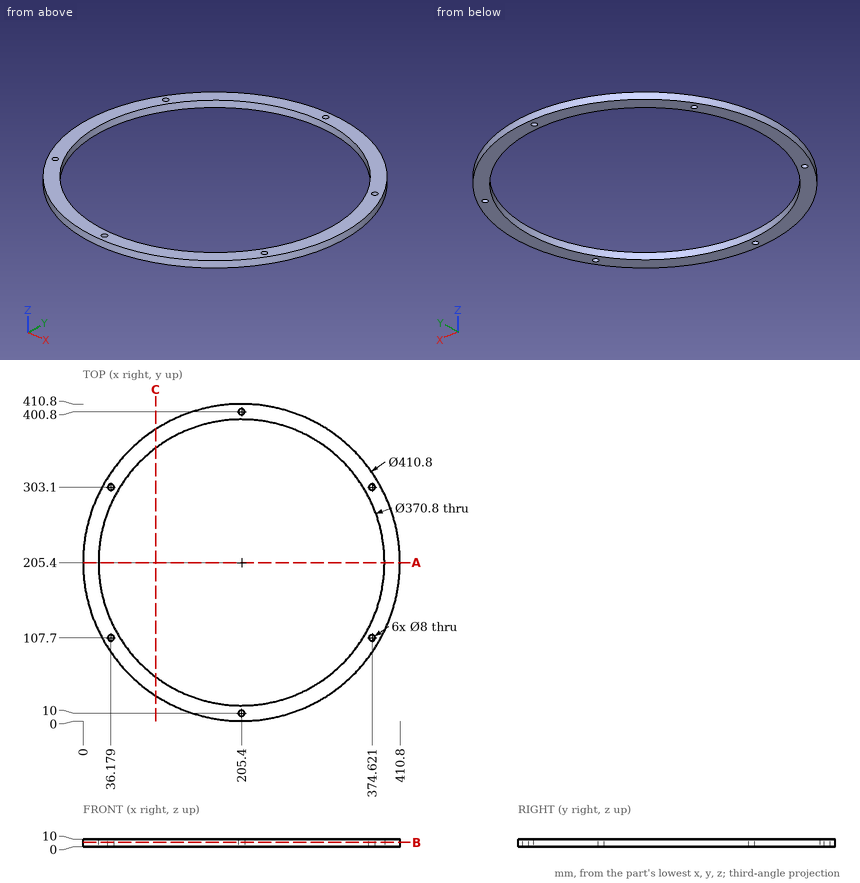
Drawing for the job (mm, zero at the part's lowest x, y, z). Round coordinates to 2 decimals unless told otherwise and drop trailing zeros. Order: outer loops, then holes, each group sorted by start corner. A loop starts at its lowest first (then second) coordinate and runs counter-clockwise, first axis right, second up. Notation, with made-up numbers: (-3.75, -15) -> (1.25, -15) arc R33 ccw to (1.25, 22) -> close; hole circle Ø10 at (15.25, 83.25). An arc over 180 degrees is marked (long way). Write item = value, one per line. Start each with the question number.
(1) Cut at B-B, the plane z = 5.5. List the corners of the cut face in (x, y).
(2) Probe line 1 (X direction, y = 108, z = 7.25) (1 decimal); line 2 (X direction, y = 303.1, z = 2.5) (1 decimal); line 3 (Y direction, x = 246, z = 8). List the from-to ranges inside material, lowest first. Write a range as [from, to].
(3) Cut at C-C, the plane x = 94. List the corners of the cut face in (y, z).
(4) Pin check, flat tips, straight feed: P1, Ø10.5, axis at x = 205.4, y = 10, coming from the -Z side; P2, Ø4, axis at y = 250.5, z = 3.5, coming from the -X side; P3, Ø1.5, axis at x = 77.5, z = 4, coming from the -Y side; P4, Ø6, axis at y = 351, z = 6.5, coming from the +X side. Stop position of each tip, or through.
(5) Cut at A-A, the plane y = 205.4. List the corners of the cut face in (x, z).
Model answer:
q1.outline = circle Ø410.8 at (205.4, 205.4); hole circle Ø370.8 at (205.4, 205.4); hole circle Ø8 at (36.18, 107.7); hole circle Ø8 at (36.18, 303.1); hole circle Ø8 at (205.4, 10); hole circle Ø8 at (205.4, 400.8); hole circle Ø8 at (374.62, 107.7); hole circle Ø8 at (374.62, 303.1)
q2.line_1 = [24.6, 32.2], [40.2, 47.6], [363.2, 370.6], [378.6, 386.2]
q2.line_2 = [24.7, 32.2], [40.2, 47.8], [363, 370.6], [378.6, 386.1]
q2.line_3 = [4.05, 24.5], [386.3, 406.75]
q3.outline = (32.83, 0) -> (57.2, 0) -> (57.2, 10) -> (32.83, 10) -> close; (353.6, 0) -> (377.97, 0) -> (377.97, 10) -> (353.6, 10) -> close
q4.P1 = 0
q4.P2 = 4.57
q4.P3 = 44.09
q4.P4 = 353.23
q5.outline = (0, 0) -> (20, 0) -> (20, 10) -> (0, 10) -> close; (390.8, 0) -> (410.8, 0) -> (410.8, 10) -> (390.8, 10) -> close
